Can you work these out from the model? Positions are in its coordinate system, mm. Face numbers are marked on the shaded views. A direction names the side the tool comes from. Give positions to 0.01 mm unless a question says otherwise; leave off trailing zeros. Write each loop counter-clockwise with the first axis right and the second up, starting at its lowest first coordinate (ties: lowest second). Pieces come first, ordered by that corner, then holes.
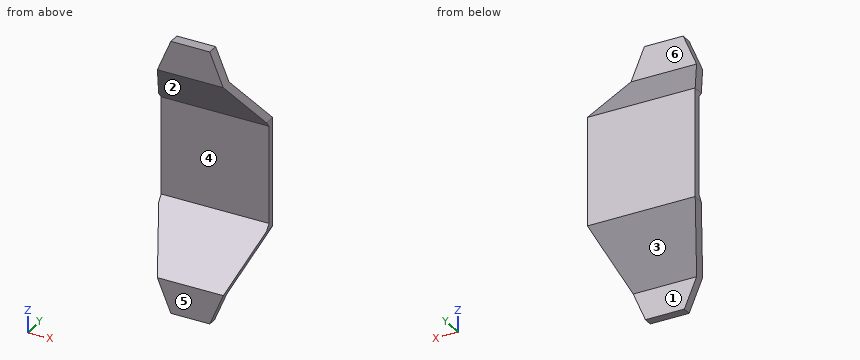
Autodesk Inventor part; units mm, degrees
ref_plane "YZ Plane" through (0, 0, 0) normal (1, 0, 0) x (0, 1, 0)
ref_plane "XZ Plane" through (0, 0, 0) normal (0, 1, 0) x (-1, 0, 0)
ref_plane "XY Plane" through (0, 0, 0) normal (0, 0, 1) x (1, 0, 0)
sketch "Эскиз1" plane through (0, 0, 0) normal (0, 1, 0) x (-1, 0, 0)
  line L0 (-25, 22.7625) -> (25, 22.7625)
  line L1 (25, 22.7625) -> (25, -22.7625)
  line L2 (25, -22.7625) -> (-25, -22.7625)
  line L3 (-25, -22.7625) -> (-25, 22.7625)
  line L4 (-25, 22.7625) -> (25, -22.7625) construction
  line L5 (25, 22.7625) -> (-25, -22.7625) construction
  point P0 (0, 0)
  dimension "d0" = 50
  dimension "d1" = 45.525
extrude "Выдавливание1" add sketch "Эскиз1" along normal blind 3
sketch "Эскиз3" plane through (25, 0, 22.7625) normal (1, 0, 0) x (0, 0, -1)
  line L0 (45.525, 0) -> (0, 0)
  line L1 (0, 0) -> (0, -21)
  line L2 (45.525, 3) -> (0, 3)
  line L3 (0, -21) -> (-43.1562, -21)
  line L4 (0, -21) -> (135.6288, -21)
  line L5 (0, 0) -> (-25.9328, -21)
  line L6 (45.525, 0) -> (71.4578, -21)
  line L7 (71.4578, -21) -> (86.4578, -21)
  line L8 (86.4578, -21) -> (86.4578, -17)
  line L9 (86.4578, -17) -> (72.8743, -17)
  line L10 (-25.9328, -21) -> (-40.9328, -21)
  line L11 (-40.9328, -21) -> (-40.9328, -16)
  line L12 (-40.9328, -16) -> (-26.1144, -16)
  line L13 (-2.6514, 3) -> (-26.1144, -16)
  line L14 (0, 3) -> (-2.6514, 3)
  line L15 (48.1764, 3) -> (72.8743, -17)
  line L16 (45.525, 3) -> (48.1764, 3)
  line L17 (0, 3) -> (0, 0)
  line L18 (45.525, 0) -> (45.525, 3)
  line L19 (45.525, 3) -> (45.525, 0)
  line L20 (45.525, 3) -> (45.525, 0)
  point P0 (22.7625, 0)
  dimension "d4" = 21
  dimension "d7" = 15
  dimension "d8" = 4
  dimension "d9" = 15
  dimension "d10" = 5
  dimension "d11" = 4
  dimension "d12" = 4
extrude "Выдавливание2" add sketch "Эскиз3" against normal up to surface (50 mm away) contours L18 L16 L15 L9 L8 L4 L6 | L5 L3 L11 L12 L13 L14 L17
sketch "Эскиз4" plane through (25, -16, 63.6953) normal (0, 1, 0) x (1, 0, 0)
  line L0 (0, 89.1092) -> (0, 38.2815)
  line L1 (0, 38.2815) -> (-16, 0)
  line L2 (0, 0) -> (-50, 0)
  line L3 (-50, 38.2815) -> (-50, 14.8184)
  line L4 (-50, 38.2815) -> (-34, 0)
  line L5 (-50, 14.8184) -> (-50, 0)
  line L6 (0, 14.8184) -> (0, 0)
  line L7 (-16, 0) -> (0, 0)
  line L8 (0, 38.2815) -> (0, 0)
  line L9 (-34, 0) -> (-50, 0)
  line L10 (-50, 0) -> (-50, 38.2815)
  point P0 (-25, 63.6953)
  dimension "d15" = 16
  dimension "d16" = 16
extrude "Выдавливание3" cut sketch "Эскиз4" along normal mid plane 70
sketch "Эскиз5" plane through (0, 3, 0) normal (0, 1, 0) x (1, 0, 0)
  line L0 (-15.1935, -48.8769) -> (-9, -63.6953)
  line L1 (-25, 25.4139) -> (-25, -25.4139)
  line L2 (-25, 25.4139) -> (-9, 63.6953)
  line L3 (25, 63.6953) -> (-25, 63.6953)
  line L4 (25, 63.6953) -> (25, 50.1118)
  line L5 (25, 25.4139) -> (9.06, 63.6953)
  line L6 (-25, 25.4139) -> (-25, 63.6953)
  line L7 (-9, 63.6953) -> (-25, 63.6953)
  line L8 (25, 25.4139) -> (25, 63.6953)
  line L9 (25, 63.6953) -> (9.06, 63.6953)
  point P0 (0, 0)
extrude "Выдавливание4" cut sketch "Эскиз5" against normal blind 70
sketch "Эскиз7" plane through (0, 3, 0) normal (0, 1, 0) x (1, 0, 0)
  line L0 (25, -25.4139) -> (-25, -25.4139)
  line L1 (25, 25.4139) -> (-25, 25.4139)
  line L2 (-25, -25.4139) -> (25, 25.4139)
  line L3 (-25, 25.4139) -> (25, -25.4139)
  line L4 (-15.65, -17.15) -> (15.65, -17.15)
  line L5 (15.65, -17.15) -> (15.65, 17.15)
  line L6 (15.65, 17.15) -> (-15.65, 17.15)
  line L7 (-15.65, 17.15) -> (-15.65, -17.15)
  line L8 (-15.65, -17.15) -> (15.65, 17.15) construction
  line L9 (15.65, -17.15) -> (-15.65, 17.15) construction
  point P0 (0, 0)
  dimension "d21" = 31.3
  dimension "d22" = 34.3
1) Suppose I cut it at C-C on y = -10. Write out the boundary of the cut face in (x, z).
Values follow:
outline: (-20.95, -35.11) - (-18.29, -41.47) - (18.32, -41.47) - (20.96, -35.11) - close; (-20.95, 35.11) - (20.95, 35.11) - (18.29, 41.47) - (-18.29, 41.47) - close
2) For the marked faces 4, 5 and 6, which set-ups out of +Z, -Z, +X, -X, +Y, -Y let a thin tool reach every point of the face, with its end or its side?
Values follow:
face 4: +X, -X, -Y
face 5: +Z, -Z, +X, -X, -Y
face 6: +Z, +X, -X, +Y
3) For pin 1 Ø2 at (x, y) = (-15, -5.5) entering from -Z; pin 2 Ø1.5 at (x, y) = (2, -6) entering from +Z; pin 3 Ø12 at (x, y) = (-14, -2) entering from -Z, each with a flat end and sliding along its axis, tell me the tip position at first contact or that it passes through.
Values follow:
pin 1: stops at z = -37.15
pin 2: stops at z = 37.45
pin 3: stops at z = -39
4) Suppose I cut it at D-D on z = -17.5. Write out the boundary of the cut face in (x, y).
Values follow:
outline: (-25, 0) - (25, 0) - (25, 3) - (-25, 3) - close
5) Please list where these lines run through material, in increasing order: L1, parallel to Z at x = 2, y = -2.5; L2, parallel to Z at x = -0.5, y = -16.5; L3, parallel to Y at x = 5.5, z = 15.5.
Values follow:
L1: z = -32.21 to -25.85, 25.85 to 32.21
L2: z = -49.49 to -43.14, 43.14 to 63.7
L3: y = 0 to 3
6) Suppose I cut it at A-A on y = -19.25. Write out the boundary of the cut face in (x, z).
Values follow:
outline: (-16.17, -46.53) - (-9, -63.7) - (9.06, -63.7) - (16.21, -46.53) - close; (-16.17, 46.53) - (16.17, 46.53) - (9, 63.7) - (-9, 63.7) - close
7) If we mould it in two halves opening along Z, with no side actions, what happens to the marked faces 1, 2 and 3? For each: +Z half, -Z half, draft (parallel to the pull), parting line (faces both ways), or undercut.
Values follow:
face 1: draft
face 2: undercut
face 3: -Z half
8) Suppose I cut it at B-B on x = 6.5. Write out the boundary of the cut face in (y, z), plus the area to 3 significant figures.
Values follow:
outline: (-21, -63.7) - (-17, -63.7) - (-17, -50.11) - (3, -25.41) - (3, 25.41) - (-16, 48.88) - (-16, 63.7) - (-21, 63.7) - (-21, 48.7) - (0, 22.76) - (0, -22.76) - (-21, -48.7) - close
area: 534 mm2
